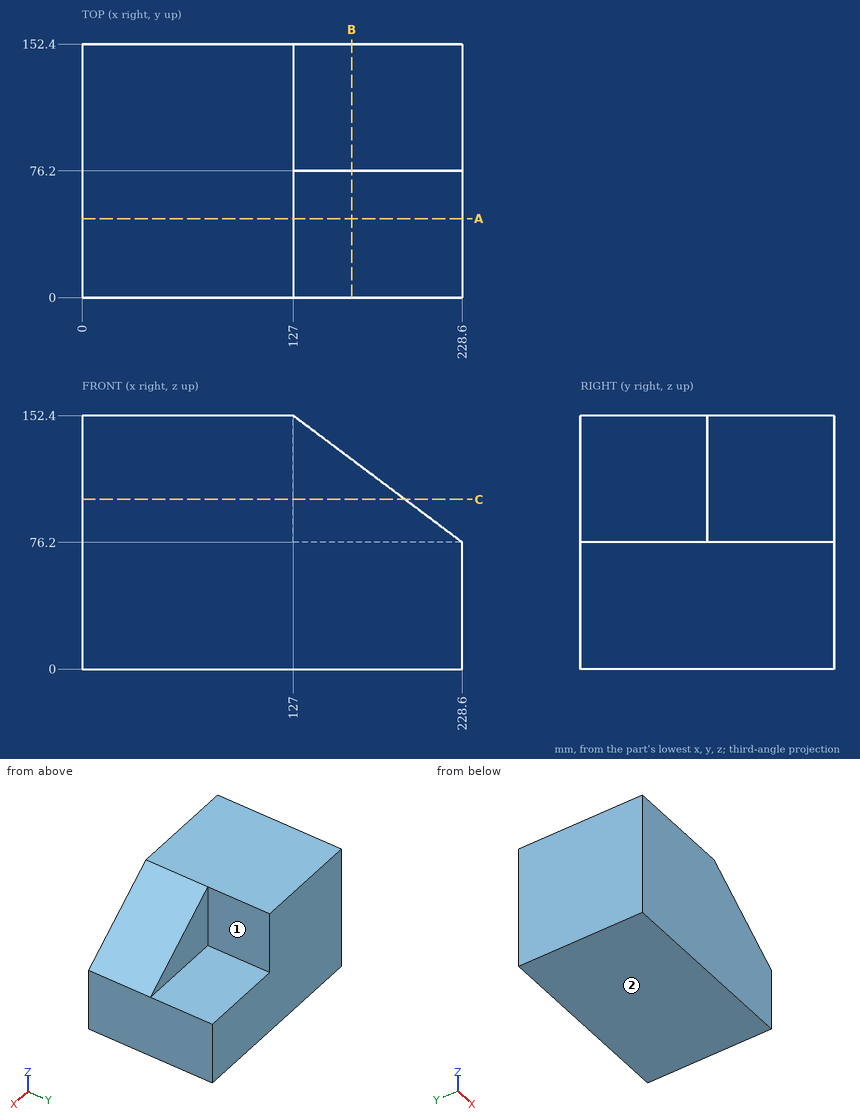
Design review of the part shown in the three views and the two pictorial views. Dimensions are in mm from the part's minimum x, y and z. A direction names the side the tool comes from. Round coordinates to 2 decimals unless told otherwise and drop trailing zeros. Order: outer loops, then holes, each group sorted by start corner. A loop starts at its lowest first (then second) coordinate and runs counter-clockwise, first axis right, second up. Notation, with made-up numbers: (5.5, -34) -> (43.5, -34) arc R20 cw to (43.5, 4) -> close; hole circle Ø7 at (17, 8.25). An arc over 180 degrees is marked (long way). Write item = value, one per line. Start each with the question number.
1) Insertion check: pin 1 (23 mm diameter, centred on y = 109, z = 106.5, fed in from +X); pin 2 (8 mm diameter, centred on y = 23.5, z = 117, fed in from +X). Each pin has a flat end and moves straight along its axis. Give the tip position at first contact, or say it passes through.
2) Take a section at B-B on x = 162. State the section outline as (y, z) points.
3) To check wall thickness, follow line 1 (Z direction, x = 160, y = 94.5); line 2 (X direction, y = 83.5, z = 132.5). State the ranges of each line that lie inside material, in increasing order. Write a range as from..to.
4) Take a section at A-A on y = 47.5. State the section outline as (x, z) points.
5) Take a section at C-C on z = 102. State the section outline as (x, y) points, plus the area to 3 significant figures.
6) Tool access review of the marked faces 1 and 2: name each direction out of +Z, -Z, +X, -X, +Y, -Y from which nothing blocks a thin tool from reaching the whole face with its end or side.
Verdict:
q1.pin_1 = 127
q1.pin_2 = 179.53
q2.outline = (0, 0) -> (152.4, 0) -> (152.4, 76.2) -> (76.2, 76.2) -> (76.2, 126.15) -> (0, 126.15) -> close
q3.line_1 = 0..76.2
q3.line_2 = 0..127
q4.outline = (0, 0) -> (228.6, 0) -> (228.6, 76.2) -> (127, 152.4) -> (0, 152.4) -> close
q5.outline = (0, 0) -> (194.2, 0) -> (194.2, 76.2) -> (127, 76.2) -> (127, 152.4) -> (0, 152.4) -> close
q5.area = 24,500 mm2
q6.face_1 = +Z, +X, +Y
q6.face_2 = -Z, +X, -X, +Y, -Y
